Source: three-view drawing plus pictorial views. Frame: mm from the lowest corner of the part. A direction names the side the tool comes from. Coordinates: 2 decimals unless noted, no trailing zeros. Order: outer loops, then holes, each group sorted by start corner. A loop starts at its lowest first (then second) coordinate and runs counter-clockwise, first axis right, second up. Notation, with made-up numbers: (46.5, 20.25) - (65.5, 20.25) arc R22 cw to (65.5, 39.25) - close; hole circle Ø8 at (39.25, 87.5). An arc over 180 degrees is marked (long way). One line per question, with ' | ' between items.
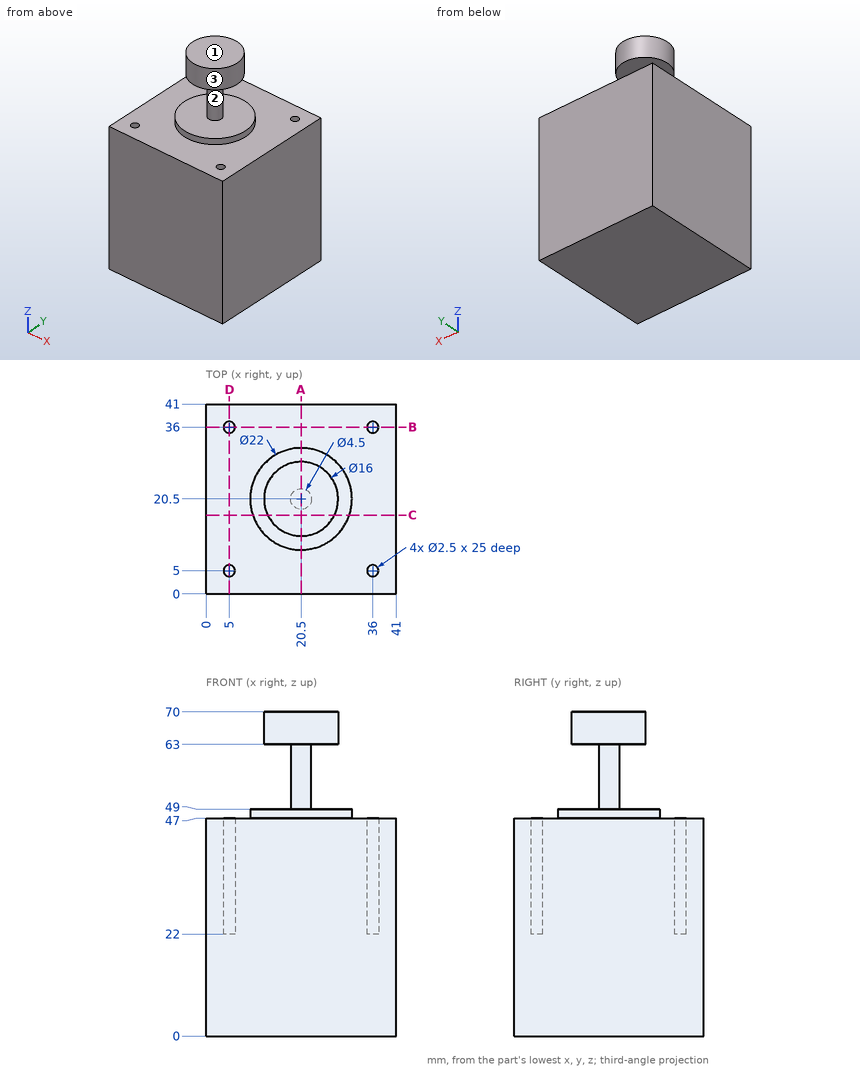
(1) Material intervals for L1, parallel to Y at x = 36, z = 40; L2, parallel to Z at x = 17.5, y = 19; L3, parallel to Z at x = 38, y = 28, sorted ascending. Write a range as from..to.
Taken from the geometry:
L1: y = 0..3.75, 6.25..34.75, 37.25..41 | L2: z = 0..49, 63..70 | L3: z = 0..47
(2) Pin query (flat end, axial travel): P1, Ø1.5, axis at x = 36, y = 36, coming from the +Z side; P2, Ø1.2, axis at x = 36.5, y = 4.5, coming from the +Z side; P3, Ø6, axis at x = 16, z = 51, coming from the -Y side. Return the tip coordinate at first contact, or that it passes through.
Taken from the geometry:
P1: stops at z = 22 | P2: stops at z = 47 | P3: stops at y = 9.74
(3) Cut plane B-B (y = 36). Return the cut outline in (x, z).
Taken from the geometry:
outline: (0, 0) - (41, 0) - (41, 47) - (37.25, 47) - (37.25, 22) - (34.75, 22) - (34.75, 47) - (6.25, 47) - (6.25, 22) - (3.75, 22) - (3.75, 47) - (0, 47) - close
(4) Set-up query: the marked faces 1, 2 and 3. Return all of +Z, -Z, +X, -X, +Y, -Y with unobstructed straight access to the full face (end or side cutting, diameter ignored); none if empty.
Taken from the geometry:
face 1: +Z, +X, -X, +Y, -Y | face 2: none | face 3: +Z
(5) Cut plane A-A (x = 20.5). Return the cut outline in (y, z).
Taken from the geometry:
outline: (0, 0) - (41, 0) - (41, 47) - (31.5, 47) - (31.5, 49) - (22.75, 49) - (22.75, 63) - (28.5, 63) - (28.5, 70) - (12.5, 70) - (12.5, 63) - (18.25, 63) - (18.25, 49) - (9.5, 49) - (9.5, 47) - (0, 47) - close
(6) Cut plane C-C (y = 17). Return the cut outline in (x, z), and give its area (3 significant figures).
Taken from the geometry:
outline: (0, 0) - (41, 0) - (41, 47) - (30.93, 47) - (30.93, 49) - (10.07, 49) - (10.07, 47) - (0, 47) - close; (13.31, 63) - (27.69, 63) - (27.69, 70) - (13.31, 70) - close | area: 2,070 mm²
